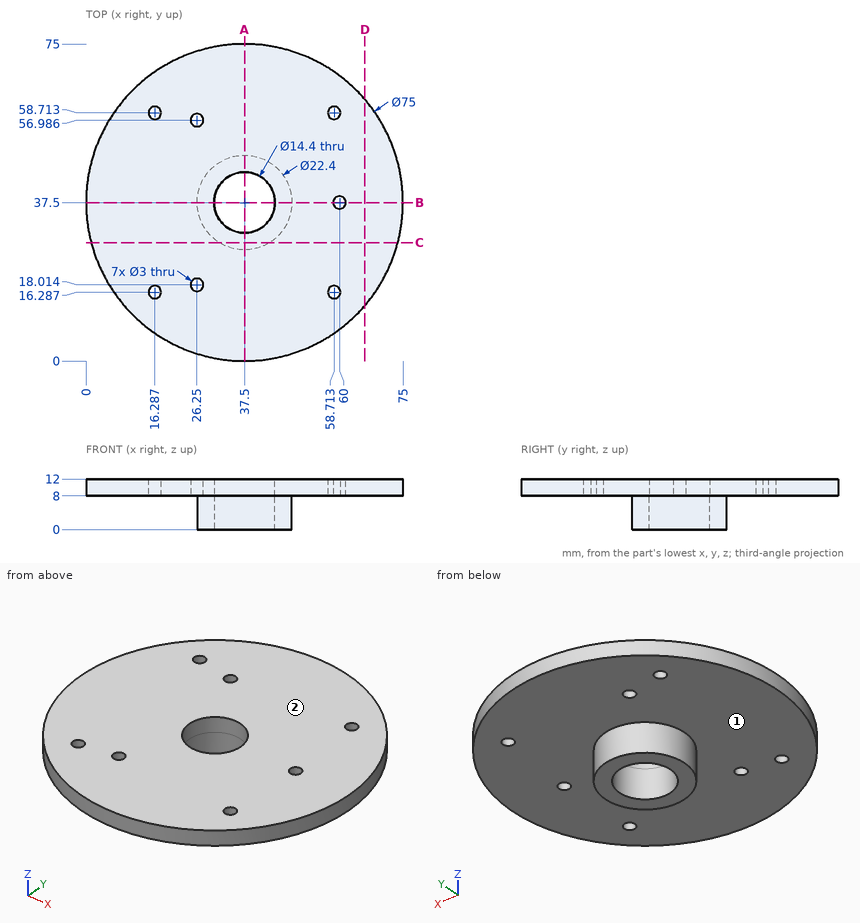
Job drawing, mm, ordinate dimensions from the low corner. One solid piece. A direction names the side the tool comes from. Round coordinates to 2 decimals unless told otherwise and drop trailing zeros. Write each loop counter-clockwise with the first axis right and the second up, starting at its lowest first coordinate (ties: lowest second). Pieces come first, ordered by that corner, then holes. Notation, with made-up numbers: M 66.25,67.5 L 103.25,67.5 A16 cw 103.25,88.5 Z; hole C -4,45.5 d5. An arc over 180 degrees is marked long. Return JSON: item names as keys, results as strings. Group by question number.
(1) Saw through at A-A on x = 37.5. Write the cut outline in (y, z).
(2) Saw through at C-C on y = 28. Write the cut outline in (x, z).
(3) Saw through at B-B on y = 37.5. Write the cut outline in (x, z).
(4) Drill centre lines: probe 1 along X at (y, z) = (60, 9.75) (1 decimal); probe 2 along Z at (x, y) = (62, 38); probe 3 along Y at (x, z) = (37.5, 9.85). Where is each one in solid material? Low to high.
(5) Pin check, flat tips, straight feed: pin 1 Ø5 at (x, y) = (14.5, 15) entering from -Z; pin 2 Ø5 at (x, z) = (42, 10) entering from +Y; pin 3 Ø6 at (y, z) = (36, 4.5) entering from -X. Stop position of each tip, or through.
(6) Saw through at D-D on x = 66. Write the cut outline in (y, z).
(7) Which spindle directions (+Z, -Z, +X, -X, +Y, -Y) get a long thin tool onto all of the face, cutting with end or side? Do the marked faces 1 and 2. Say none if no direction does.
Returned:
{
 "1": {"outline": "M 0,8 L 26.3,8 L 26.3,0 L 30.3,0 L 30.3,12 L 0,12 Z; M 44.7,0 L 48.7,0 L 48.7,8 L 75,8 L 75,12 L 44.7,12 Z"},
 "2": {"outline": "M 1.22,8 L 31.57,8 L 31.57,0 L 43.43,0 L 43.43,8 L 73.78,8 L 73.78,12 L 1.22,12 Z"},
 "3": {"outline": "M 0,8 L 26.3,8 L 26.3,0 L 30.3,0 L 30.3,12 L 0,12 Z; M 44.7,0 L 48.7,0 L 48.7,8 L 58.5,8 L 58.5,12 L 44.7,12 Z; M 61.5,8 L 75,8 L 75,12 L 61.5,12 Z"},
 "4": {"probe 1": "7.5 to 15.5, 17.1 to 57.9, 59.5 to 67.5", "probe 2": "8 to 12", "probe 3": "0 to 30.3, 44.7 to 75"},
 "5": {"pin 1": "z = 8", "pin 2": "y = 74.95", "pin 3": "x = 26.3"},
 "6": {"outline": "M 13.13,8 L 61.87,8 L 61.87,12 L 13.13,12 Z"},
 "7": {"face 1": "-Z", "face 2": "+Z, +X, -X, +Y, -Y"}
}
